Verification items for the finished model (mm, model axes). Face numbers are marked on the shaded views. Coordinates: 2 decimals unless noted, no trailing zeros. Loops run counter-clockwise (first coordinate to the right, second up) from the corner with the lowest first, then second, coordinate; pieces in that order, holes last. Notation, with made-up numbers: (-35.5, 66) - (-29.5, 66) arc R23 ccw to (-29.5, 84) - close; hole circle Ø7 at (-20, 18.5). An arc over 180 degrees is marked (long way). Answer as CSV lines item,"result". Start each with the question number.
1. Cross-section at A-A (z = 0). Enter the section's corners in (x, y), plus the area to 3 significant figures.
2. Release check for a two-part mould opening along Z. For the marked faces 1, 2 and 3 record: pulls with the +Z half, pulls with the -Z half, needs draft (parallel to the pull), parting line crosses it, or undercut.
3. Material ranges on line 1 (X direction, y = -14.55, z = 0); line 2 (X direction, y = -19.3, z = 0); line 3 (X direction, y = -15.5, z = 6.25), recorded low to high. Write a range as [from, to].
4. Cross-section at B-B (x = 12). Enter the section's corners in (y, z).
5. Gauge pin test, flat ends, axial feed: P1, Ø8, axis at y = -8, z = 9, coming from the -X side; P2, Ø1.5, axis at y = 0, z = 3.5, coming from the -X side; P3, Ø4, axis at x = 8.5, y = 4, coming from the -Z side; P4, Ø13, axis at x = 13.5, z = -2, coming from the -Y side. Record the tip position at first contact, or that the pin passes through.
6. Cross-section at D-D (x = 1.75). Enter the section's corners in (y, z), plus the area to 3 significant figures.
7. Cross-section at C-C (y = -9.5). Enter the section's corners in (x, z), plus the area to 3 significant figures.
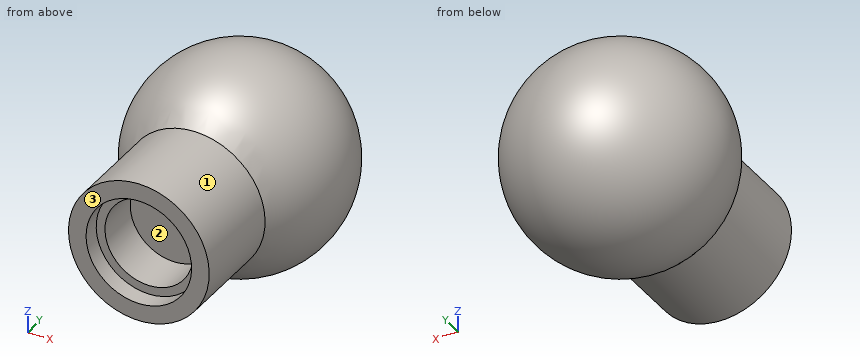
```python
from build123d import *

# Parameters (mm, degrees)
BOSS_EXTRUDE1_REACH      = 52.706
BOSS_EXTRUDE1_END_RADIUS = 12
BOSS_EXTRUDE1_START      = 5
SKETCH3_R                = 8
SKETCH4_R                = 6
CUT_EXTRUDE2_DEPTH       = 2
SKETCH5_R                = 5
CUT_EXTRUDE3_DEPTH       = 5


with BuildPart() as part:
    # Sketch2 → Revolve1 (revolve)
    with BuildSketch(Plane(origin=(0, 0, 0), x_dir=(1, 0, 0), z_dir=(0, 1, 0))):
        with BuildLine():
            Line((0, 0), (24, 0))
            ThreePointArc((24, 0), (12, 12), (0, 0))
        make_face()
    revolve(axis=Axis((0, 0, 0), (1, 0, 0)))

    # Boss-Extrude1: up to this sphere (the profile starts outside it)
    boss_extrude1_end = Location((12, 0, 0)) * Sphere(BOSS_EXTRUDE1_END_RADIUS, mode=Mode.PRIVATE)
    # Sketch3 → Boss-Extrude1 (add, up to the surface)
    with BuildSketch(Plane(origin=(0, -25, 0), x_dir=(1, 0, 0), z_dir=(0, 1, 0)).offset(BOSS_EXTRUDE1_START), mode=Mode.PRIVATE) as boss_extrude1_sk1:
        with Locations(Location((12, 0, 0), (0, 0, 270))):
            Circle(SKETCH3_R)
    boss_extrude1_tool1 = extrude(boss_extrude1_sk1.sketch, amount=BOSS_EXTRUDE1_REACH, mode=Mode.PRIVATE) - boss_extrude1_end
    add(boss_extrude1_tool1.solids().sort_by_distance((12, -20, 0))[0])

    # Sketch4 → Cut-Extrude2 (cut)
    with BuildSketch(Plane.XZ.offset(20)):
        with Locations(Location((12, 0, 0), (0, 0, 270))):
            Circle(SKETCH4_R)
    extrude(amount=-CUT_EXTRUDE2_DEPTH, mode=Mode.SUBTRACT)

    # Sketch5 → Cut-Extrude3 (cut)
    with BuildSketch(Plane.XZ.offset(18)):
        with Locations(Location((12, 0, 0), (0, 0, 270))):
            Circle(SKETCH5_R)
    extrude(amount=-CUT_EXTRUDE3_DEPTH, mode=Mode.SUBTRACT)


solid = part.part
```
Values follow:
1,outline,"(4, -20) - (6, -20) - (6, -18) - (7, -18) - (7, -13) - (17, -13) - (17, -18) - (18, -18) - (18, -20) - (20, -20) - (20, -8.94) arc R12 ccw (long way) to (4, -8.94) - close"
1,area,"522 mm²"
2,face 1,"parting line crosses it"
2,face 2,"undercut"
2,face 3,"needs draft"
3,line 1,"x = [4, 7], [17, 20]"
3,line 2,"x = [4, 6], [18, 20]"
3,line 3,"x = [7.01, 16.99]"
4,outline,"(-20, -8) - (-8.94, -8) arc R12 ccw (long way) to (-8.94, 8) - (-20, 8) - (-20, 6) - (-18, 6) - (-18, 5) - (-13, 5) - (-13, -5) - (-18, -5) - (-18, -6) - (-20, -6) - close"
5,P1,"stops at x = 3.09"
5,P2,"stops at x = 0.32"
5,P3,"stops at z = -11.53"
5,P4,"stops at y = -20"
6,outline,"circle Ø12.48 at (0, 0)"
6,area,"122 mm²"
7,outline,"circle Ø16 at (12, 0)"
7,area,"201 mm²"
